Autodesk Inventor part; units mm, degrees
ref_plane "YZ Plane" through (0, 0, 0) normal (1, 0, 0) x (0, 1, 0)
ref_plane "XZ Plane" through (0, 0, 0) normal (0, 1, 0) x (-1, 0, 0)
ref_plane "XY Plane" through (0, 0, 0) normal (0, 0, 1) x (1, 0, 0)
sketch "Sketch1" plane through (0, 0, 0) normal (0, 1, 0) x (-1, 0, 0)
  circle A0 centre (0, 0) radius 13.97
  line L0 (-19.05, 19.05) -> (19.05, 19.05)
  line L1 (19.05, 19.05) -> (19.05, -19.05)
  line L2 (19.05, -19.05) -> (-19.05, -19.05)
  line L3 (-19.05, -19.05) -> (-19.05, 19.05)
  line L4 (-19.05, 19.05) -> (19.05, -19.05) construction
  line L5 (19.05, 19.05) -> (-19.05, -19.05) construction
  dimension "d0" = 27.94
  dimension "d1" = 38.1
  dimension "d2" = 38.1
extrude "Extrusion1" add sketch "Sketch1" along normal blind 5.08
sketch "Sketch2" plane through (0, 5.08, 0) normal (0, 1, 0) x (1, 0, 0)
  circle A0 centre (0, 0) radius 13.97 construction
  line L0 (-19.05, -19.05) -> (-19.05, 19.05) construction
  line L1 (-19.05, 19.05) -> (19.05, 19.05) construction
  line L2 (19.05, 19.05) -> (19.05, -19.05) construction
  line L3 (19.05, -19.05) -> (-19.05, -19.05) construction
  line L4 (-19.05, -19.05) -> (0, 0) construction
  point P0 (-13.97, -13.97)
  point P1 (13.97, -13.97)
  point P2 (13.97, 13.97)
  point P3 (-13.97, 13.97)
  dimension "d5" = 13.97
  dimension "d8" = 360
hole "Hole1" at (-13.97, 5.08, 13.97) at (13.97, 5.08, 13.97) at (13.97, 5.08, -13.97) at (-13.97, 5.08, -13.97) direction (0, -1, 0) diameter 5 end through all
fillet "Fillet1" radius 3.175 4 edges at (-19.05, 2.54, 19.05) (-19.05, 2.54, -19.05) (19.05, 2.54, -19.05) (19.05, 2.54, 19.05)
equation "\"d2\" = d1"
properties part number "BearingMount" material "Wood (Birch)"
Geometry check sheet. Reference: the model listing, model coordinates, mm. Round coordinates to 2 decimals unless told otherwise and drop trailing zeros. Write each loop counter-clockwise with the first axis right and the second up, starting at its lowest first coordinate (ties: lowest second). Pieces come first, ordered by that corner, then holes. Notation, with made-up numbers: (10.25, 24.5) - (45.25, 24.5) arc R16 ccw to (45.25, 44.5) - close; hole circle Ø5 at (66, 7.5). An arc over 180 degrees is marked (long way). One line per item, written item: value.
1. Mould release check, pull along X, two halves, no side actions. Record for faces 1 (the face through (0, 3, 19.05)), 2 (the face through (19.05, 3, 0)), 3 (the face through (-16.08, 2.5, -12.63)), 4 (the face through (1.82, 2.5, -13.85)): released by +X, released by -X, zero draft, split by the parting line, or undercut.
The answers:
face 1: zero draft
face 2: released by +X
face 3: undercut
face 4: undercut
2. Cross-section at B-B on y = 1.1. Record the boundary of the cut face in (x, z) (3 decimals).
The answers:
outline: (-19.05, -15.875) arc R3.175 ccw to (-15.875, -19.05) - (15.875, -19.05) arc R3.175 ccw to (19.05, -15.875) - (19.05, 15.875) arc R3.175 ccw to (15.875, 19.05) - (-15.875, 19.05) arc R3.175 ccw to (-19.05, 15.875) - close; hole circle Ø5 at (-13.97, -13.97); hole circle Ø5 at (-13.97, 13.97); hole circle Ø27.94 at (0, 0); hole circle Ø5 at (13.97, -13.97); hole circle Ø5 at (13.97, 13.97)
3. Cross-section at A-A on z = 0. Record the boundary of the cut face in (x, y), and give its area (3 significant figures).
The answers:
outline: (-19.05, 0) - (-13.97, 0) - (-13.97, 5.08) - (-19.05, 5.08) - close; (13.97, 0) - (19.05, 0) - (19.05, 5.08) - (13.97, 5.08) - close
area: 51.6 mm^2
4. Depth check by flat-ended pin: pin 1 Ø3 at (x, z) = (13.97, 13.97) entering from +Y. Enter the tip coordinate at first touch or a pass-through.
The answers:
pin 1: passes through
5. Cross-section at D-D on z = -15. Record the boundary of the cut face in (x, y).
The answers:
outline: (-19.05, 0) - (-16.25, 0) - (-16.25, 5.08) - (-19.05, 5.08) - close; (-11.69, 0) - (11.69, 0) - (11.69, 5.08) - (-11.69, 5.08) - close; (16.25, 0) - (19.05, 0) - (19.05, 5.08) - (16.25, 5.08) - close
6. Cross-section at C-C on x = 0. Record the boundary of the cut face in (y, z).
The answers:
outline: (0, -19.05) - (5.08, -19.05) - (5.08, -13.97) - (0, -13.97) - close; (0, 13.97) - (5.08, 13.97) - (5.08, 19.05) - (0, 19.05) - close
7. Scan lines: L1, parallel to X at y = 4.15, z = 14; L2, parallel to Z at x = 0, y = 3.6; L3, parallel to X at y = 4.25, z = 0.5. Record each from-to range of solid material in increasing order.
The answers:
L1: x = -19.05 to -16.47, -11.47 to 11.47, 16.47 to 19.05
L2: z = -19.05 to -13.97, 13.97 to 19.05
L3: x = -19.05 to -13.96, 13.96 to 19.05
